from build123d import *

# Parameters (mm, degrees)
F0_R     = 25
F1_DEPTH = 100
F3_DEPTH = 50
F4_R     = 20


with BuildPart() as f1:
    # F0 (on Top) → F1 (new body)
    with BuildSketch(Plane.XY):
        with BuildLine():
            Line((200, 37.5), (0, 37.5))
            ThreePointArc((0, 37.5), (-30.618622, -21.650635), (35.355339, -12.5))
            ThreePointArc((35.355339, -12.5), (40.837221, -5.252551), (49.497475, -2.5))
            Line((49.497475, -2.5), (200, -2.5))
            Line((200, -2.5), (200, 37.5))
        make_face()
        Circle(F0_R, mode=Mode.SUBTRACT)
    extrude(amount=F1_DEPTH)

    # F2 (on face) → F3 (cut)
    with BuildSketch(Plane.XZ.offset(2.5)):
        with BuildLine():
            Line((200, 67.5), (77.039003, 67.5))
            ThreePointArc((77.039003, 67.5), (59.539003, 50), (77.039003, 32.5))
            Line((77.039003, 32.5), (200, 32.5))
            Line((200, 32.5), (200, 67.5))
        make_face()
    extrude(amount=-F3_DEPTH, mode=Mode.SUBTRACT)

    # F4
    f4_edges = [f1.edges().sort_by_distance(p)[0] for p in [
        (200, 17.5, 100),
        (200, 17.5, 0),
    ]]
    fillet(f4_edges, radius=F4_R)


solid = f1.part
Could you check a few things on this model? Use its own coordinates, in mm. A direction names the side the tool comes from. Give positions to 0.01 mm unless a question says otherwise; leave off trailing zeros. Order: outer loops, then holes, each group sorted by start corner. A loop starts at its lowest first (then second) coordinate and runs counter-clockwise, first axis right, second up. Notation, with made-up numbers: (67, 27) - (85, 27) arc R29 cw to (85, 55) - close; hole circle Ø1 at (11, 41). An arc over 180 degrees is marked (long way). One line per question, with ' | ' between items. Start each with the question number.
Item 1: For faces 5 (the cylindrical face through (193.986, 17.78, 5.703)), 6 (the flat face through (124, -2.5, 72)), 7 (the flat face through (138, 17, 32.5)), which set-ups out of +Z, -Z, +X, -X, +Y, -Y let a thin tool reach every point of the face, with its end or its side?
Item 2: I want a section at B-B on x = -12.5. Write out the boundary of the cut face in (y, z).
Item 3: I want a section at C-C on z = 76.5. Write out the boundary of the cut face in (x, y), then the cut area to 3 significant figures.
Item 4: I want a section at D-D on y = 32. Write out the boundary of the cut face in (x, z).
Item 5: Thinking about a two-plate mould opening in Y: for faces 1 (the flat face through (101, 37.5, 72)), 2 (the cylindrical face through (23.846, 7.509, 49.3)), 3 (the flat face through (70, 9, 100)), 4 (the cylindrical face through (40.73, -5.33, 49.3)), which applies, pulls with the +Y half, pulls with the -Y half, needs draft (parallel to the pull), parting line crosses it, or undercut?
Item 6: I want a section at A-A on y = 0. Write out the boundary of the cut face in (x, z), then the cut area to 3 significant figures.
Item 7: I'm going to push flat-ended pins straight in: pin 1 Ø2 at (y, z) = (-25.5, 34.5) entering from +X; pin 2 Ø12 at (y, z) = (-12, 75.5) entering from +X. Where does each tip first touch, or does it pass through?
Item 8: I need wall thicknesses on probe 1 along Z at (x, y) = (170.5, 19); probe 2 along Y at (x, z) = (0, 46); probe 3 along Y at (x, z) = (63, 74). Which ranges of each line are inside material? Lowest first, please. Write a range as [from, to].
Verdict:
1) face 5: -Z, +X, +Y, -Y | face 6: +Z, -Z, +X, -Y | face 7: +X, +Y, -Y
2) outline: (-35.36, 0) - (-21.65, 0) - (-21.65, 100) - (-35.36, 100) - close; (21.65, 0) - (35.36, 0) - (35.36, 100) - (21.65, 100) - close
3) outline: (0, 37.5) arc R37.5 ccw (long way) to (35.36, -12.5) arc R15 cw to (49.5, -2.5) - (200, -2.5) - (200, 37.5) - close; hole circle Ø50 at (0, 0) | area: 9,280 mm^2
4) outline: (-19.55, 0) - (180, 0) arc R20 ccw to (200, 20) - (200, 32.5) - (77.04, 32.5) arc R17.5 cw to (77.04, 67.5) - (200, 67.5) - (200, 80) arc R20 ccw to (180, 100) - (-19.55, 100) - close
5) face 1: pulls with the +Y half | face 2: undercut | face 3: needs draft | face 4: pulls with the -Y half
6) outline: (-37.5, 0) - (-25, 0) - (-25, 100) - (-37.5, 100) - close; (25, 0) - (180, 0) arc R20 ccw to (200, 20) - (200, 32.5) - (77.04, 32.5) arc R17.5 cw to (77.04, 67.5) - (200, 67.5) - (200, 80) arc R20 ccw to (180, 100) - (25, 100) - close | area: 13,800 mm^2
7) pin 1: x = 28.39 | pin 2: x = 39.87
8) probe 1: [0, 32.5], [67.5, 100] | probe 2: [-37.5, -25], [25, 37.5] | probe 3: [-2.5, 37.5]
